Geometry: see drawing. Coordinates: mm, zero at the bounding-box minimum. A direction names the side the tool comes from. Coordinates: 2 decimals unless noted, no trailing zeros. Order: outer loops, then holes, each group sorted by start corner. A loop starts at its lowest first (then second) coordinate and runs counter-clockwise, first axis right, second up. Notation, with made-up numbers: (-23, 32) -> (24, 32) arc R21 cw to (24, 42) -> close; hole circle Ø7 at (33, 79). An arc over 180 degrees is marked (long way). Use CSV: the item, a comma, the result in double quotes. Start each with the question number.
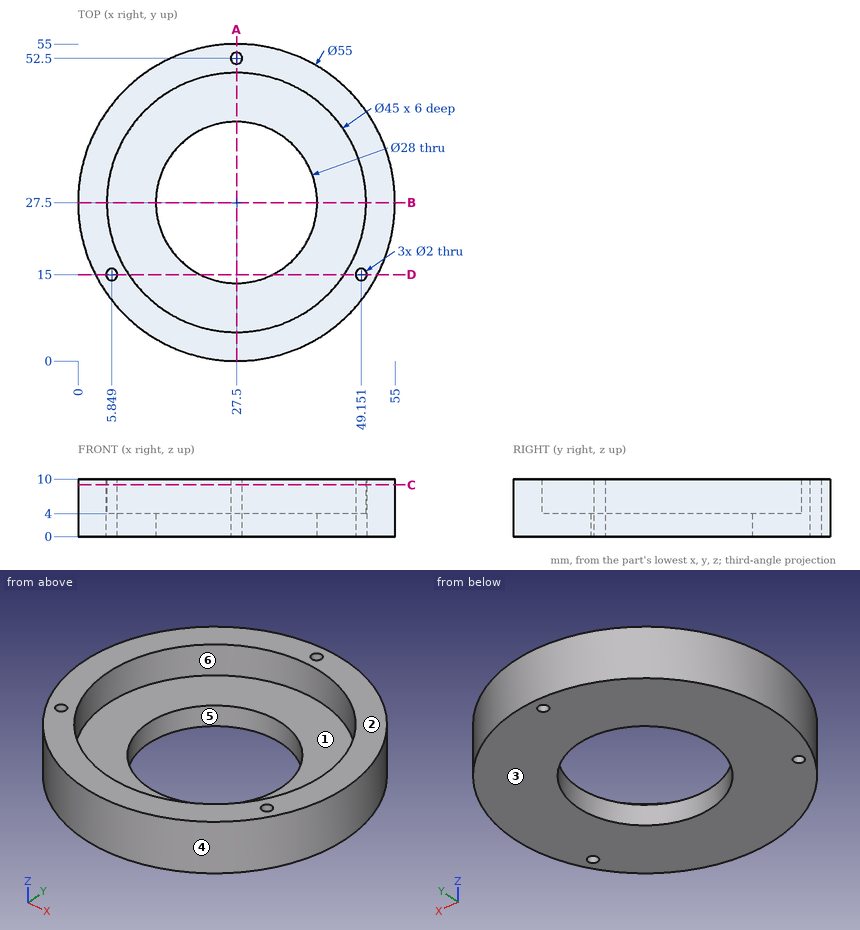
(1) Access query for the marked faces 1 and 2. Directions: +Z, -Z, +X, -X, +Y, -Y. A direction counts if a zero-diameter tool reaches every point of the face in a straight line with its end or side. Return the directions, or none.
(2) Section A-A (x = 27.5). Return loops of the section in (y, z).
(3) Section B-B (y = 27.5). Return loops of the section in (x, z).
(4) Mould query, pull axis Y, two halves, no side actions, for the marked faces 3, 4, 5 and 6. Classes: pulls with the +Y half, pulls with the -Y half, needs draft (parallel to the pull), parting line crosses it, or undercut.
(5) Section D-D (y = 15). State how many separate pieces and enclosed holes the cut face has, then the cut area to 3 significant figures.
(6) Section C-C (z = 9). Return loops of the section in (x, y).
(7) First-contact query: pin 1 (4 mm diameter, centred on x = 33.5, y = 17, fed in from +Z); pin 2 (6 mm diameter, centred on y = 40, z = 1, fed in from +X); pin 3 (4 mm diameter, centred on x = 23, z = 8, fed in from +Y); pin 4 (10 mm diameter, centred on x = 26, y = 33.5, fed in from -Z). Flat tips, straight axial feed; report the tip coordinate or a pass-through.
(8) Line query: line 1 (Y direction, x = 27.5, z = 4.25); line 2 (Y direction, x = 27.5, z = 1.95); line 3 (X direction, y = 15.5, z = 4.5) (1 decimal). Output: solid intervals per line, ascending. Write a range as from..to.
Check sheet entries:
1,face 1,"+Z"
1,face 2,"+Z, +X, -X, +Y, -Y"
2,outline,"(0, 0) -> (13.5, 0) -> (13.5, 4) -> (5, 4) -> (5, 10) -> (0, 10) -> close; (41.5, 0) -> (51.5, 0) -> (51.5, 10) -> (50, 10) -> (50, 4) -> (41.5, 4) -> close; (53.5, 0) -> (55, 0) -> (55, 10) -> (53.5, 10) -> close"
3,outline,"(0, 0) -> (13.5, 0) -> (13.5, 4) -> (5, 4) -> (5, 10) -> (0, 10) -> close; (41.5, 0) -> (55, 0) -> (55, 10) -> (50, 10) -> (50, 4) -> (41.5, 4) -> close"
4,face 3,"needs draft"
4,face 4,"parting line crosses it"
4,face 5,"undercut"
4,face 6,"undercut"
5,separate pieces,"4"
5,enclosed holes,"0"
5,area,"175 mm^2"
6,outline,"circle Ø55 at (27.5, 27.5); hole circle Ø2 at (5.85, 15); hole circle Ø45 at (27.5, 27.5); hole circle Ø2 at (27.5, 52.5); hole circle Ø2 at (49.15, 15)"
7,pin 1,"stops at z = 4"
7,pin 2,"stops at x = 53.31"
7,pin 3,"stops at y = 54.89"
7,pin 4,"passes through"
8,line 1,"y = 0..5, 50..51.5, 53.5..55"
8,line 2,"y = 0..13.5, 41.5..51.5, 53.5..55"
8,line 3,"x = 2.8..5, 6.7..8.5, 46.5..48.3, 50..52.2"
